The listing builds one solid part. Answer for the finished solid, in the listing's coordinates (mm). A direction names the side the tool comes from. Coordinates: 2 decimals unless noted, no trailing zeros. Write each loop counter-clockwise with the first axis right and the second up, starting at its lowest first coordinate (ties: lowest second). Pieces come first, ordered by that corner, then holes.
(1) The part is cut by section C-C on x = 26. Determine the outline of the cut face in (y, z), plus the area to 3 significant figures.
(2) For a pull along Z with two mould halves and no side action, classify faces 4 (the flat face through (-0.791, -1.986, 11.215)), 5 (the flat face through (0.539, -1.972, 12.124)), 6 (the flat face through (-0.791, -3.493, -8.578)), 7 (the flat face through (47.374, -3.3, 1.7)) as +Z half, -Z half, draft (parallel to the pull), parting line (faces both ways), or undercut.
(3) Which of the six approach directions +Z, -Z, +X, -X, +Y, -Y give full straight-line access (tool end or side, diameter ignored) to faces 1 (the flat face through (-1, -4, 2)), 2 (the flat face through (-11, -3, 2)), 3 (the flat face through (-0.791, -1.479, -8.376))?
(4) The part is cut by section B-B on z = 0.5. Determine the outline of the cut face in (x, y), plus the area to 3 significant figures.
(5) The part is cut by section D-D on x = 5.5. Determine the outline of the cut face in (y, z).
(6) Straight lines are drawn through the part: line 1 (Y direction, x = -18.5, z = 4); line 2 (Z direction, x = -6, y = -1.85); line 3 (Z direction, x = -4, y = -1.5). For each, find the intervals that lie inside material, in ascending order.
(7) The part is cut by section A-A on y = -2.15. Determine the outline of the cut face in (x, z), plus the area to 3 significant figures.
from build123d import *

# Parameters (mm, degrees)
F1_DEPTH = 1
F3_DEPTH = 2
F5_DEPTH = 1


with BuildPart() as f1:
    # F0 (on Front) → F1 (new body)
    with BuildSketch(Plane.XZ):
        Polygon((47.37426, 8.919068), (-47.62574, 15.419068), (-47.62574, -11.580932), (47.37426, -5.080932), align=None)
    extrude(amount=F1_DEPTH)

    # F2 (on face) → F3 (join)
    with BuildSketch(Plane.XZ.offset(1)):
        Polygon((47.37426, 8.919068), (-47.62574, 15.419068), (-47.62574, 14.419068), (47.37426, 7.919068), align=None)
        Polygon((-47.62574, -10.580932), (-47.62574, -11.580932), (47.37426, -5.080932), (47.37426, -4.080932), align=None)
    extrude(amount=F3_DEPTH)

    # F4 (on face) → F5 (join)
    with BuildSketch(Plane.XZ.offset(3)):
        Polygon((47.37426, 8.919068), (-47.62574, 15.419068), (-47.62574, -11.753376), (47.37426, -5.31239), align=None)
    extrude(amount=F5_DEPTH)


solid = f1.part
Model answer:
1. outline: (-4, -6.76) - (-3, -6.76) - (-3, -6.54) - (0, -6.54) - (0, 10.38) - (-4, 10.38) - close; hole (-3, -5.54) - (-1, -5.54) - (-1, 9.38) - (-3, 9.38) - close
1. area: 38.1 mm2
2. face 4: undercut
2. face 5: +Z half
2. face 6: -Z half
2. face 7: draft
3. face 1: +Z, -Z, +X, -X, -Y
3. face 2: -X
3. face 3: -Z, +X, +Y
4. outline: (-47.63, -4) - (47.37, -4) - (47.37, -3) - (-47.63, -3) - close; (-47.63, -1) - (47.37, -1) - (47.37, 0) - (-47.63, 0) - close
4. area: 190 mm2
5. outline: (-4, -8.15) - (-3, -8.15) - (-3, -7.95) - (0, -7.95) - (0, 11.78) - (-4, 11.78) - close; hole (-3, -6.95) - (-1, -6.95) - (-1, 10.78) - (-3, 10.78) - close
6. line 1: y = -4 to -3, -1 to 0
6. line 2: z = -8.73 to -7.73, 11.57 to 12.57
6. line 3: z = -8.6 to -7.6, 11.43 to 12.43
7. outline: (-47.63, -11.58) - (47.37, -5.08) - (47.37, -4.08) - (-47.63, -10.58) - close; (-47.63, 14.42) - (47.37, 7.92) - (47.37, 8.92) - (-47.63, 15.42) - close
7. area: 190 mm2
